```python
from build123d import *

# Parameters (mm, degrees)
SKETCH_1_W          = 20
SKETCH_1_H          = 20
SKETCH_1_R          = 2.1
EXTRUDE_1_DEPTH     = 10
SKETCH_2_W          = 20
SKETCH_2_H          = 10
EXTRUDE_2_DEPTH     = 5
SKETCH_3_W          = 20
SKETCH_3_H          = 5
EXTRUDE_3_DEPTH     = 25
SKETCH_4_R          = 2.1
CUT_EXTRUDE_1_DEPTH = 25


with BuildPart() as part:
    # 草图1 → 凸台-拉伸1 (new body)
    with BuildSketch(Plane.XY):
        Rectangle(SKETCH_1_W, SKETCH_1_H)
        with Locations((0, 5.2)):
            Circle(SKETCH_1_R, mode=Mode.SUBTRACT)
        with Locations((0, -5.2)):
            Circle(SKETCH_1_R, mode=Mode.SUBTRACT)
    extrude(amount=EXTRUDE_1_DEPTH)

    # 草图2 → 凸台-拉伸2 (add)
    with BuildSketch(Plane(origin=(0, 10, 0), x_dir=(1, 0, 0), z_dir=(0, 1, 0))):
        with Locations((0, -5)):
            Rectangle(SKETCH_2_W, SKETCH_2_H)
    extrude(amount=EXTRUDE_2_DEPTH)

    # 草图3 → 凸台-拉伸3 (add)
    with BuildSketch(Plane.XY.offset(10)):
        with Locations((0, 12.5)):
            Rectangle(SKETCH_3_W, SKETCH_3_H)
    extrude(amount=EXTRUDE_3_DEPTH)

    # 草图4 → 切除-拉伸1 (cut)
    with BuildSketch(Plane.XZ.offset(-10)):
        with Locations((-6, 31)):
            Circle(SKETCH_4_R)
        with Locations((6, 31)):
            Circle(SKETCH_4_R)
    extrude(amount=-CUT_EXTRUDE_1_DEPTH, mode=Mode.SUBTRACT)


solid = part.part
```
Geometry check sheet. Reference: the model listing, model coordinates, mm. A direction names the side the tool comes from. Coordinates: 2 decimals unless noted, no trailing zeros. Order: outer loops, then holes, each group sorted by start corner. A loop starts at its lowest first (then second) coordinate and runs counter-clockwise, first axis right, second up.
Q1. Sectioned sample at D-D on x = 0. Record the cut outline in (y, z).
Reply:
outline: (-10, 0) - (-7.3, 0) - (-7.3, 10) - (-10, 10) - close; (-3.1, 0) - (3.1, 0) - (3.1, 10) - (-3.1, 10) - close; (7.3, 0) - (15, 0) - (15, 35) - (10, 35) - (10, 10) - (7.3, 10) - close
Q2. Depth check by flat-ended pin: pin 1 Ø12 at (x, z) = (-1.5, 17.5) entering from -Y; pin 2 Ø2 at (x, y) = (-3.5, 6.5) entering from +Z. Enter the tip coordinate at first touch or a pass-through.
Reply:
pin 1: stops at y = 10
pin 2: stops at z = 10
Q3. Sectioned sample at C-C on y = -5.2. Record the cut outline in (x, z), and give its area (3 significant figures).
Reply:
outline: (-10, 0) - (-2.1, 0) - (-2.1, 10) - (-10, 10) - close; (2.1, 0) - (10, 0) - (10, 10) - (2.1, 10) - close
area: 158 mm2
Q4. Tool access check on faces 1 (the face through (-6.46, 12.46, 28.95)), 2 (the face through (0, 0, 10)). Record the directions out of +Z, -Z, +X, -X, +Y, -Y that give a thin tool (end or side, any length) a straight path to the whole face; none if there is none.
Reply:
face 1: +Y, -Y
face 2: +Z, +X, -X, -Y
Q5. Sectioned sample at B-B on z = 31. Record the cut outline in (x, y).
Reply:
outline: (-10, 10) - (-8.1, 10) - (-8.1, 15) - (-10, 15) - close; (-3.9, 10) - (3.9, 10) - (3.9, 15) - (-3.9, 15) - close; (8.1, 10) - (10, 10) - (10, 15) - (8.1, 15) - close
Q6. Thickness scan on probe 1 along Y at (x, z) = (0.25, 2); probe 2 along Z at (x, y) = (6, 13.5); probe 3 along Y at (x, z) = (0.25, 17). Record the ranges inside material, lowest first.
Reply:
probe 1: y = -10 to -7.29, -3.11 to 3.11, 7.29 to 15
probe 2: z = 0 to 28.9, 33.1 to 35
probe 3: y = 10 to 15
Q7. Sectioned sample at A-A on x = 6. Record the cut outline in (y, z), and give its area (3 significant figures).
Reply:
outline: (-10, 0) - (15, 0) - (15, 28.9) - (10, 28.9) - (10, 10) - (-10, 10) - close; (10, 33.1) - (15, 33.1) - (15, 35) - (10, 35) - close
area: 354 mm2
Q8. Draft check along X on faces 3 (the face through (5.54, 12.46, 28.95)), 4 (the face through (0, 15, 17)), 5 (the face through (-10, 5, 9)). Enter one of: released by +X, released by -X, zero draft, split by the parting line, or undercut.
Reply:
face 3: undercut
face 4: zero draft
face 5: released by -X
